from build123d import *

# Parameters (mm, degrees)
BOSS_EXTRUDE1_DEPTH = 30
SHELL1_T            = -3
BOSS_EXTRUDE2_DEPTH = 8
SKETCH2_R           = 8.5
CUT_EXTRUDE1_DEPTH  = 6.5
SKETCH5_R           = 6
CUT_EXTRUDE4_DEPTH  = 13
BOSS_EXTRUDE3_START = 5
SKETCH6_R           = 9
SKETCH6_R_2         = 6
BOSS_EXTRUDE3_DEPTH = 5
SKETCH7_R           = 4
CUT_EXTRUDE5_DEPTH  = 7
BOSS_EXTRUDE4_START = 5
SKETCH7_3_R         = 6
SKETCH7_3_R_2       = 4
BOSS_EXTRUDE4_DEPTH = 5
SKETCH8_R           = 1.5
CUT_EXTRUDE6_DEPTH  = 221.884585248
SKETCH9_R           = 3
CUT_EXTRUDE7_DEPTH  = 3


with BuildPart() as part:
    # Sketch1 → Boss-Extrude1 (new body)
    with BuildSketch(Plane(origin=(0, 0, 0), x_dir=(1, 0, 0), z_dir=(0, 1, 0))):
        with BuildLine():
            ThreePointArc((-36, 0), (0, -36), (36, 0))
            Line((36, 0), (36, 66))
            Line((36, 66), (-36, 66))
            Line((-36, 66), (-36, 0))
        make_face()
    extrude(amount=-BOSS_EXTRUDE1_DEPTH)

    # Shell1
    shell1_openings = [part.faces().sort_by_distance(p)[0] for p in [
        (0, -15, -66),
    ]]
    offset(amount=SHELL1_T, openings=shell1_openings, kind=Kind.INTERSECTION)

    # Sketch1_3 → Boss-Extrude2 (add)
    with BuildSketch(Plane(origin=(0, 0, 0), x_dir=(1, 0, 0), z_dir=(0, 1, 0))):
        with BuildLine():
            Line((-70, 206), (70, 206))
            ThreePointArc((70, 206), (73.535533906, 204.535533906), (75, 201))
            Line((75, 201), (75, 71))
            ThreePointArc((75, 71), (73.535533906, 67.464466094), (70, 66))
            Line((70, 66), (-70, 66))
            ThreePointArc((-70, 66), (-73.535533906, 67.464466094), (-75, 71))
            Line((-75, 71), (-75, 201))
            ThreePointArc((-75, 201), (-73.535533906, 204.535533906), (-70, 206))
        make_face()
    extrude(amount=-BOSS_EXTRUDE2_DEPTH)

    # Sketch2 → Cut-Extrude1 (cut)
    with BuildSketch(Plane.XZ.offset(30)):
        with Locations(Location((13, -10.3, 0), (0, 0, 270))):
            Circle(SKETCH2_R)
        with Locations(Location((-13, -10.3, 0), (0, 0, 270))):
            Circle(SKETCH2_R)
    extrude(amount=-CUT_EXTRUDE1_DEPTH, mode=Mode.SUBTRACT)

    # Sketch5 → Cut-Extrude4 (cut)
    with BuildSketch(Plane.XZ.offset(30)):
        with Locations(Location((0, 8, 0), (0, 0, 270))):
            Circle(SKETCH5_R)
    extrude(amount=-CUT_EXTRUDE4_DEPTH, mode=Mode.SUBTRACT)

    # Sketch6 → Boss-Extrude3 (add)
    with BuildSketch(Plane.XZ.offset(30).offset(BOSS_EXTRUDE3_START)):
        with Locations(Location((0, 8, 0), (0, 0, 270))):
            Circle(SKETCH6_R)
        with Locations(Location((0, 8, 0), (0, 0, 270))):
            Circle(SKETCH6_R_2, mode=Mode.SUBTRACT)
    extrude(amount=-BOSS_EXTRUDE3_DEPTH)

    # Sketch7 → Cut-Extrude5 (cut)
    with BuildSketch(Plane.XZ.offset(30)):
        with Locations(Location((0, 24, 0), (0, 0, 270))):
            Circle(SKETCH7_R)
    extrude(amount=-CUT_EXTRUDE5_DEPTH, mode=Mode.SUBTRACT)

    # Sketch7_3 → Boss-Extrude4 (add)
    with BuildSketch(Plane.XZ.offset(30).offset(BOSS_EXTRUDE4_START)):
        with Locations(Location((0, 24, 0), (0, 0, 90))):
            Circle(SKETCH7_3_R)
        with Locations(Location((0, 24, 0), (0, 0, 270))):
            Circle(SKETCH7_3_R_2, mode=Mode.SUBTRACT)
    extrude(amount=-BOSS_EXTRUDE4_DEPTH)

    # Sketch8 → Cut-Extrude6 (cut, through all)
    with BuildSketch(Plane.XZ.offset(8)):
        with Locations(Location((68, -73, 0), (0, 0, 270))):
            Circle(SKETCH8_R)
        with Locations(Location((68, -199, 0), (0, 0, 270))):
            Circle(SKETCH8_R)
        with Locations(Location((-68, -199, 0), (0, 0, 270))):
            Circle(SKETCH8_R)
        with Locations(Location((-68, -73, 0), (0, 0, 270))):
            Circle(SKETCH8_R)
    extrude(amount=-CUT_EXTRUDE6_DEPTH, mode=Mode.SUBTRACT)

    # Sketch9 → Cut-Extrude7 (cut)
    with BuildSketch(Plane(origin=(0, 0, 0), x_dir=(1, 0, 0), z_dir=(0, 1, 0))):
        with Locations(Location((-68, 73, 0), (0, 0, 270))):
            Circle(SKETCH9_R)
        with Locations(Location((-68, 199, 0), (0, 0, 270))):
            Circle(SKETCH9_R)
        with Locations(Location((68, 199, 0), (0, 0, 270))):
            Circle(SKETCH9_R)
        with Locations(Location((68, 73, 0), (0, 0, 270))):
            Circle(SKETCH9_R)
    extrude(amount=-CUT_EXTRUDE7_DEPTH, mode=Mode.SUBTRACT)


solid = part.part
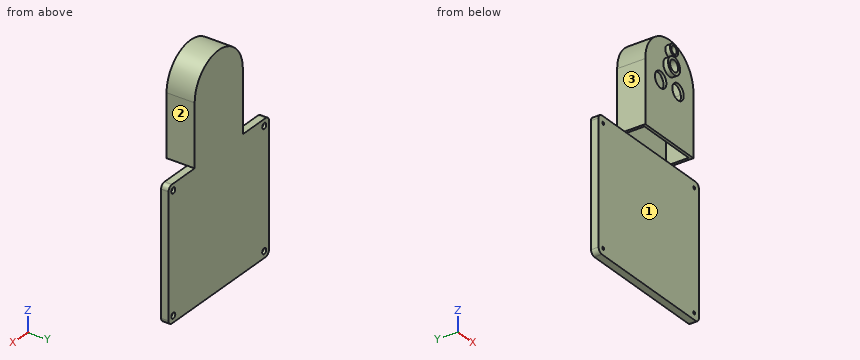
Source: CAD feature listing. Evaluate the final solid. Frame: model axes, mm. Face numbers are marked on the shaded views. A direction names the side the tool comes from. Round coordinates to 2 decimals unless told otherwise and drop trailing zeros. Loops run counter-clockwise (first coordinate to the right, second up) from the corner with the lowest first, then second, coordinate; pieces in that order, holes last. Notation, with made-up numbers: M 25,78 L 38,78 A20 ccw 38,117 Z; hole C -33.5,22 d8. An arc over 180 degrees is marked long. Return JSON: item names as keys, results as strings. Group by question number.
1. Section query D-D on x = 18. Output: boundary loops of the cut face in (y, z), and give its area (3 significant figures).
2. Section query C-C on y = -16.5. Output: boundary loops of the cut face in (x, z), and give its area (3 significant figures).
3. Pin query (flat end, axial travel): pin 1 (12 mm diameter, centred on x = -39, z = -6.5, fed in from -Y); pin 2 (9.5 mm diameter, centred on x = 0, z = 8, fed in from -Y); pin 3 (19 mm diameter, centred on y = -12.5, z = -19, fed in from +X). Return the tip coordinate at first contact, or that it passes through.
4. Section query A-A on x = -13. Output: boundary loops of the cut face in (y, z), and give its area (3 significant figures).
5. Reachability of the marked faces 1, 2 and 3 from +Z, -Z, +X, -X, +Y, -Y: full face, straight path, thin tool, end or side. Return the list, or none.
6. Section query B-B on z = -57. Output: boundary loops of the cut face in (x, y), and give its area (3 significant figures).
7. Material intervals for line 1 along Z through (x, y) = (-68, -6.8); line 2 along X through (y, z) = (-5.3, -73); line 3 along X through (y, z) = (-28.3, -10.3), sorted ascending. Write a range as from..to.
Checks:
{
 "1": {"outline": "M -30,-66 L -27,-66 L -27,-17.17 L -30,-17.17 Z; M -30,-3.43 L -27,-3.43 L -27,27.66 L -3,27.66 L -3,-66 L -8,-66 L -8,-206 L 0,-206 L 0,31.18 L -30,31.18 Z", "area": "1,750 mm²"},
 "2": {"outline": "M -36,-66 L -33,-66 L -33,0 A33 cw 33,0 L 33,-66 L 36,-66 L 36,0 A36 ccw -36,0 Z", "area": "721 mm²"},
 "3": {"pin 1": "stops at y = -30", "pin 2": "stops at y = -3", "pin 3": "stops at x = 36"},
 "4": {"outline": "M -30,-66 L -27,-66 L -27,-18.8 L -30,-18.8 Z; M -30,-1.8 L -27,-1.8 L -27,30.33 L -3,30.33 L -3,-66 L -8,-66 L -8,-206 L 0,-206 L 0,33.57 L -30,33.57 Z", "area": "1,740 mm²"},
 "5": {"face 1": "-Z, +X, -X, -Y", "face 2": "+Z, +X, +Y, -Y", "face 3": "+Z, -X, +Y, -Y"},
 "6": {"outline": "M -36,-30 L 36,-30 L 36,0 L -36,0 Z; hole M -33,-27 L 33,-27 L 33,-3 L -33,-3 Z", "area": "576 mm²"},
 "7": {"line 1": "z = -206..-200.5, -197.5..-74.5, -71.5..-66", "line 2": "x = -75..-69.5, -66.5..66.5, 69.5..75", "line 3": "x = -36..-21.5, -4.5..4.5, 21.5..36"}
}
